from build123d import *

# Parameters (mm, degrees)
SKETCH_1_R          = 8
SKETCH_1_R_2        = 1.6
EXTRUDE_1_DEPTH     = 1.5
FILLET_1_R          = 1
SKETCH_3_R          = 2.25
CUT_EXTRUDE_3_DEPTH = 0.4
FILLET_2_R          = 0.4


with BuildPart() as part:
    # Эскиз1 → Бобышка-Вытянуть1 (new body)
    with BuildSketch(Plane.XY):
        Circle(SKETCH_1_R)
        Circle(SKETCH_1_R_2, mode=Mode.SUBTRACT)
    extrude(amount=EXTRUDE_1_DEPTH)

    # Скругление1
    fillet_1_edges = [part.edges().sort_by_distance(p)[0] for p in [
        (-8, 0, 1.5),
    ]]
    fillet(fillet_1_edges, radius=FILLET_1_R)

    # Эскиз3 → Вырез-Вытянуть3 (cut)
    with BuildSketch(Plane.XY.offset(1.5)):
        Circle(SKETCH_3_R)
    extrude(amount=-CUT_EXTRUDE_3_DEPTH, mode=Mode.SUBTRACT)

    # Скругление2
    fillet_2_edges = [part.edges().sort_by_distance(p)[0] for p in [
        (-2.25, 0, 1.5),
    ]]
    fillet(fillet_2_edges, radius=FILLET_2_R - 0.0001)  # a hair under: the kernel refuses the full size


solid = part.part
Build history of the part. All positions in model axes, mm. Round coordinates to 2 decimals unless told otherwise and drop trailing zeros. Write each loop counter-clockwise with the first axis right and the second up, starting at its lowest first coordinate (ties: lowest second). Pieces come first, ordered by that corner, then holes. Notation, with made-up numbers: M -22.75,35.5 L -9.75,35.5 A20 cw -9.75,44.5 Z; hole C -26.5,89 d2. An arc over 180 degrees is marked long. Use CSV: the item, a comma, the result in double quotes.
1. Wall check: probe 1 along Y at (x, z) = (0, 0.45); probe 2 along X at (y, z) = (1.5, 1.15); probe 3 along Y at (x, z) = (0, 1.15). Give the ranges that are in metal, low to high. Write a range as from..to.
Reply:
probe 1,"y = -8..-1.6, 1.6..8"
probe 2,"x = -7.61..-1.68, 1.68..7.61"
probe 3,"y = -7.76..-2.25, 2.25..7.76"
2. Saw through at C-C (z = 1.3). Give the cut face in (x, y), plus the area to 3 significant figures.
Reply:
outline,"C 0,0 d15.2; hole C 0,0 d4.61"
area,"165 mm²"
3. Flat gauge pin, fed straight in: pin 1 (2.5 mm diameter, centred on x = 0, y = 0, fed in from +Z). Where does the tip first touch, or does it go through?
Reply:
pin 1,"passes through"
4. Two-plate mould, pull along Y, no slides. Class faces 1 (the face through (-1.27, -0.97, 0.54)), 2 (the face through (-1.73, -7.81, 0.25)), 3 (the face through (-2, 0, 1.1)), 4 (the face through (0, -3, 1.5)): +Y half, -Y half, draft (parallel to the pull), parting line (faces both ways), or undercut.
Reply:
face 1,"undercut"
face 2,"parting line"
face 3,"undercut"
face 4,"draft"
5. Saw through at D-D (z = 0.2). Give the cut face in (x, y), plus the area to 3 significant figures.
Reply:
outline,"C 0,0 d16; hole C 0,0 d3.2"
area,"193 mm²"
